from build123d import *

# Parameters (mm, degrees)
EXTRUDE_1_DEPTH     = 1500
SKETCH_2_R          = 2.5
CUT_EXTRUDE_1_DEPTH = 61
SKETCH_3_R          = 2.5
CUT_EXTRUDE_2_DEPTH = 61


with BuildPart() as part:
    # Эскиз1 → Вытянуть-Тонкостенный1 (new body)
    with BuildSketch(Plane(origin=(0, 0, 0), x_dir=(1, 0, 0), z_dir=(0, 1, 0))):
        Polygon((0, 60), (0, 0), (60, 0), (60, 2), (2, 2), (2, 60), align=None)
    extrude(amount=EXTRUDE_1_DEPTH)

    # Эскиз2 → Вырез-Вытянуть1 (cut, through all)
    with BuildSketch(Plane.ZY):
        with Locations((-18.5, 30)):
            Circle(SKETCH_2_R)
        with Locations((-18.5, 80)):
            Circle(SKETCH_2_R)
        with Locations((-18.5, 130)):
            Circle(SKETCH_2_R)
        with Locations((-18.5, 180)):
            Circle(SKETCH_2_R)
        with Locations((-18.5, 230)):
            Circle(SKETCH_2_R)
        with Locations((-18.5, 280)):
            Circle(SKETCH_2_R)
        with Locations((-18.5, 330)):
            Circle(SKETCH_2_R)
        with Locations((-18.5, 380)):
            Circle(SKETCH_2_R)
        with Locations((-18.5, 430)):
            Circle(SKETCH_2_R)
        with Locations((-18.5, 480)):
            Circle(SKETCH_2_R)
        with Locations((-18.5, 530)):
            Circle(SKETCH_2_R)
        with Locations((-18.5, 580)):
            Circle(SKETCH_2_R)
        with Locations((-18.5, 630)):
            Circle(SKETCH_2_R)
        with Locations((-18.5, 680)):
            Circle(SKETCH_2_R)
        with Locations((-18.5, 730)):
            Circle(SKETCH_2_R)
        with Locations((-18.5, 780)):
            Circle(SKETCH_2_R)
        with Locations((-18.5, 830)):
            Circle(SKETCH_2_R)
        with Locations((-18.5, 880)):
            Circle(SKETCH_2_R)
        with Locations((-18.5, 930)):
            Circle(SKETCH_2_R)
        with Locations((-18.5, 980)):
            Circle(SKETCH_2_R)
        with Locations((-18.5, 1030)):
            Circle(SKETCH_2_R)
        with Locations((-18.5, 1080)):
            Circle(SKETCH_2_R)
        with Locations((-18.5, 1130)):
            Circle(SKETCH_2_R)
        with Locations((-18.5, 1180)):
            Circle(SKETCH_2_R)
        with Locations((-18.5, 1230)):
            Circle(SKETCH_2_R)
        with Locations((-18.5, 1280)):
            Circle(SKETCH_2_R)
        with Locations((-18.5, 1330)):
            Circle(SKETCH_2_R)
        with Locations((-18.5, 1380)):
            Circle(SKETCH_2_R)
        with Locations((-18.5, 1430)):
            Circle(SKETCH_2_R)
        with Locations((-18.5, 1480)):
            Circle(SKETCH_2_R)
    extrude(amount=-CUT_EXTRUDE_1_DEPTH, mode=Mode.SUBTRACT)

    # Эскиз3 → Вырез-Вытянуть2 (cut, through all)
    with BuildSketch(Plane.XY):
        with Locations((18.5, 30)):
            Circle(SKETCH_3_R)
        with Locations((18.5, 80)):
            Circle(SKETCH_3_R)
        with Locations((18.5, 130)):
            Circle(SKETCH_3_R)
        with Locations((18.5, 180)):
            Circle(SKETCH_3_R)
        with Locations((18.5, 230)):
            Circle(SKETCH_3_R)
        with Locations((18.5, 280)):
            Circle(SKETCH_3_R)
        with Locations((18.5, 330)):
            Circle(SKETCH_3_R)
        with Locations((18.5, 380)):
            Circle(SKETCH_3_R)
        with Locations((18.5, 430)):
            Circle(SKETCH_3_R)
        with Locations((18.5, 480)):
            Circle(SKETCH_3_R)
        with Locations((18.5, 530)):
            Circle(SKETCH_3_R)
        with Locations((18.5, 580)):
            Circle(SKETCH_3_R)
        with Locations((18.5, 630)):
            Circle(SKETCH_3_R)
        with Locations((18.5, 680)):
            Circle(SKETCH_3_R)
        with Locations((18.5, 730)):
            Circle(SKETCH_3_R)
        with Locations((18.5, 780)):
            Circle(SKETCH_3_R)
        with Locations((18.5, 830)):
            Circle(SKETCH_3_R)
        with Locations((18.5, 880)):
            Circle(SKETCH_3_R)
        with Locations((18.5, 930)):
            Circle(SKETCH_3_R)
        with Locations((18.5, 980)):
            Circle(SKETCH_3_R)
        with Locations((18.5, 1030)):
            Circle(SKETCH_3_R)
        with Locations((18.5, 1080)):
            Circle(SKETCH_3_R)
        with Locations((18.5, 1130)):
            Circle(SKETCH_3_R)
        with Locations((18.5, 1180)):
            Circle(SKETCH_3_R)
        with Locations((18.5, 1230)):
            Circle(SKETCH_3_R)
        with Locations((18.5, 1280)):
            Circle(SKETCH_3_R)
        with Locations((18.5, 1330)):
            Circle(SKETCH_3_R)
        with Locations((18.5, 1380)):
            Circle(SKETCH_3_R)
        with Locations((18.5, 1430)):
            Circle(SKETCH_3_R)
        with Locations((18.5, 1480)):
            Circle(SKETCH_3_R)
    extrude(amount=-CUT_EXTRUDE_2_DEPTH, mode=Mode.SUBTRACT)


solid = part.part
Work out the finished part from the listing and answer in its coordinate system (mm). A direction names the side the tool comes from. Round coordinates to 2 decimals unless told otherwise and drop trailing zeros. Write each loop counter-clockwise with the first axis right and the second up, starting at its lowest first coordinate (ties: lowest second). Pieces come first, ordered by that corner, then holes. Notation, with made-up numbers: (-23.75, -35) - (-5.75, -35) arc R14 ccw to (-5.75, -20) - close; hole circle Ø10 at (81, 50). An arc over 180 degrees is marked (long way). Answer in a Markdown table with one row per item. Add a question column.
1. Find the intervals of material crossed by line 1 along Z through (x, y) = (0.85, 380); line 2 along X through (y, z) = (780, -0.5); line 3 along X through (y, z) = (146, -55.5), in increasing order. Write a range as from..to.
2. For faces 1 (the flat face through (2, 740, -31)), 2 (the flat face through (0, 740, -30)), determine the directions among +Z, -Z, +X, -X, +Y, -Y from which every point of the face is accessible in a straight line to the end or side of a thin tool.
3. Given pin 1 (6 mm diameter, centred on y = 1256, z = -44, fed in from -X); pin 2 (4.5 mm diameter, centred on y = 80, z = -18.5, fed in from +X); pin 3 (6.5 mm diameter, centred on y = 1130, z = -18.5, fed in from +X); pin 4 (6.5 mm diameter, centred on x = 18.5, y = 380, fed in from -Z), each flat-ended and moving along its own axis, determine where each tip first touches the part or whether it passes through.
4. A cutting plane is placed at B-B, the plane z = -50.5. Determine the outline of the cut face in (x, y).
5. A cutting plane is placed at A-A, the plane y = 854.5. Determine the outline of the cut face in (x, z), and give its area (3 significant figures).
Worked out:
| question | item | result |
|---|---|---|
| 1 | line 1 | -60..-21, -16..0 |
| 1 | line 2 | 0..16, 21..60 |
| 1 | line 3 | 0..2 |
| 2 | face 1 | -Z, +X, +Y, -Y |
| 2 | face 2 | +Z, -Z, -X, +Y, -Y |
| 3 | pin 1 | x = 0 |
| 3 | pin 2 | through |
| 3 | pin 3 | x = 2 |
| 3 | pin 4 | z = -2 |
| 4 | outline | (0, 0) - (2, 0) - (2, 1500) - (0, 1500) - close |
| 5 | outline | (0, -60) - (2, -60) - (2, -2) - (60, -2) - (60, 0) - (0, 0) - close |
| 5 | area | 236 mm^2 |
